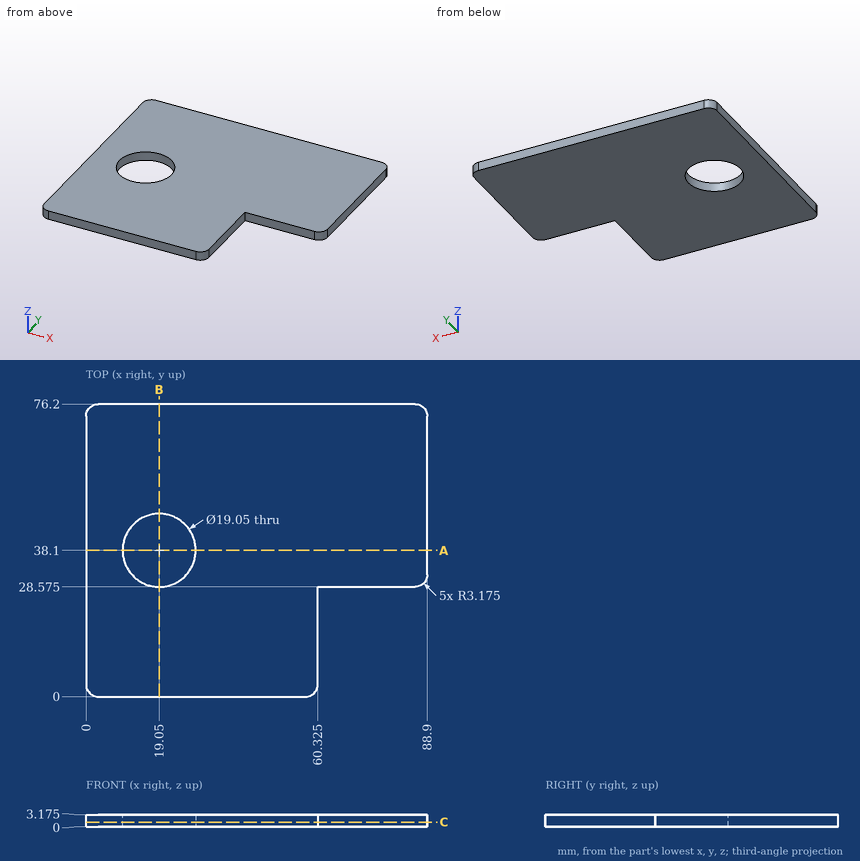
Source: three-view drawing plus pictorial views. Frame: mm from the lowest corner of the part. Give positions to 0.01 mm unless a question says otherwise; leave off trailing zeros. Order: outer loops, then holes, each group sorted by start corner. A loop starts at its lowest first (then second) coordinate and runs counter-clockwise, first axis right, second up. Notation, with made-up numbers: M 14,78 L 36,78 A12 ccw 36,91 Z; hole C -21.5,71.5 d5. An arc over 180 degrees is marked long. Return JSON: item names as keys, results as strings.
1) Contact query for a flat-ended pin moving along its axis: pin 1 (11.5 mm diameter, centred on x = 19.05, y = 38.1, fed in from -Z). Output: stop coordinate, or through.
Taken from the geometry:
{"pin 1": "passes through"}
2) Section query C-C on z = 1.2. Output: boundary loops of the cut face in (x, y) (3 decimals).
Taken from the geometry:
{"outline": "M 0,3.175 A3.175 ccw 3.175,0 L 57.15,0 A3.175 ccw 60.325,3.175 L 60.325,28.575 L 85.725,28.575 A3.175 ccw 88.9,31.75 L 88.9,73.025 A3.175 ccw 85.725,76.2 L 3.175,76.2 A3.175 ccw 0,73.025 Z; hole C 19.05,38.1 d19.05"}
3) Section query B-B on x = 19.05. Output: boundary loops of the cut face in (y, z) (3 decimals), and give its area (3 significant figures).
Taken from the geometry:
{"outline": "M 0,0 L 28.575,0 L 28.575,3.175 L 0,3.175 Z; M 47.625,0 L 76.2,0 L 76.2,3.175 L 47.625,3.175 Z", "area": "181 mm2"}
4) Line query: L1, parallel to Y at x = 19.05, z = 1.6 (3 decimals); L2, parallel to X at y = 44.5, z = 2.25; L3, parallel to Y at x = 66, z = 3.05 (3 decimals). Output: solid intervals per line, ascending. Write a range as [from, to].
Taken from the geometry:
{"L1": "y = [0, 28.575], [47.625, 76.2]", "L2": "x = [0, 12], [26.1, 88.9]", "L3": "y = [28.575, 76.2]"}
5) Section query A-A on y = 38.1. Output: boundary loops of the cut face in (x, z) (3 decimals), and give its area (3 significant figures).
Taken from the geometry:
{"outline": "M 0,0 L 9.525,0 L 9.525,3.175 L 0,3.175 Z; M 28.575,0 L 88.9,0 L 88.9,3.175 L 28.575,3.175 Z", "area": "222 mm2"}
